Can you work these out from the drawing? Everything is in mm from the part's minimum corner. A direction names the side the tool comes from. Coordinates: 2 decimals unless noted, no trailing zeros. Loops run counter-clockwise (first coordinate to the right, second up) from the corner with the lowest first, then second, coordinate; pieces in that order, holes last.
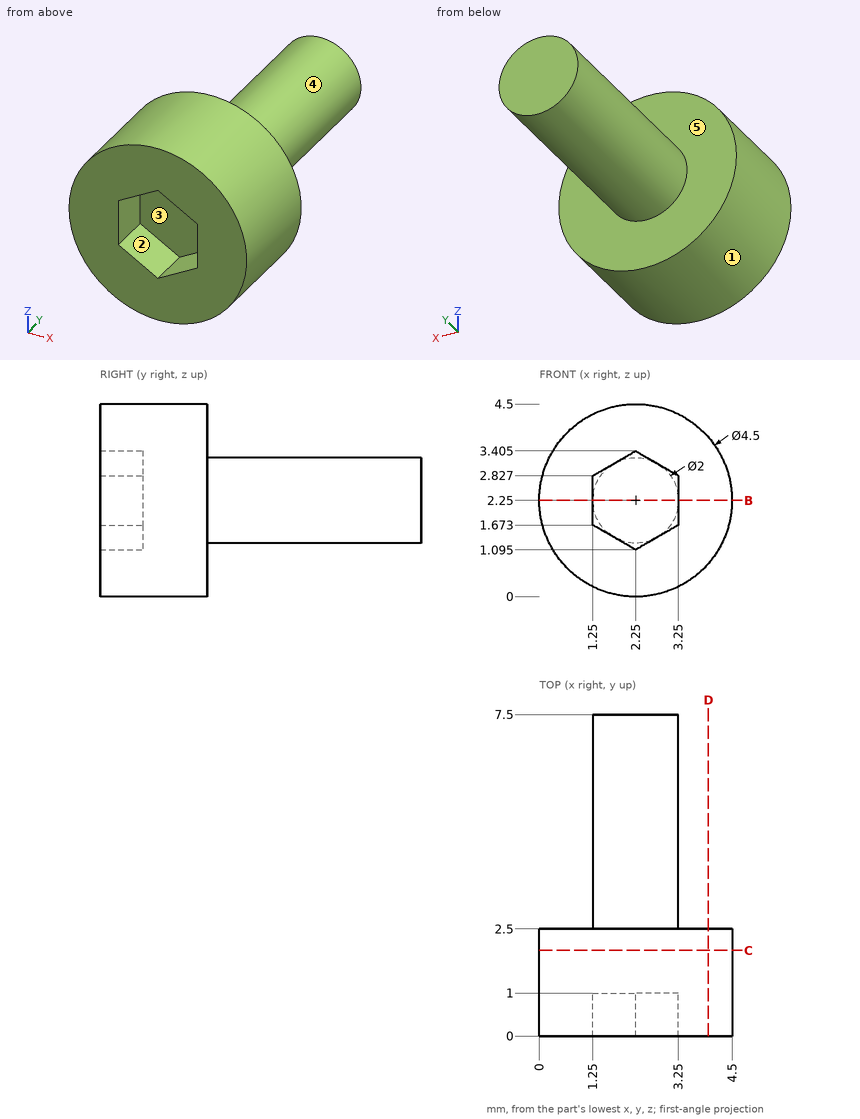
1. I want a section at D-D (x = 3.95). Please give me the cut outline in (y, z).
2. On a 3-axis mill with a long thin cutter (end or side, diameter ignored), from which of +Z, -Z, +X, -X, +Y, -Y can I reach the whole of each face in a straight line? I mean the marked faces 1 and 2. Say none if no direction works.
3. I want a section at B-B (z = 2.25). Please give me the cut outline in (x, y).
4. I want a section at C-C (y = 2). Please give me the cut outline in (x, z).
5. We'd pull the mould along Z, two halves only. Please class the marked faces 3, 4 and 5: +Z half, -Z half, draft (parallel to the pull), parting line (faces both ways), or undercut.
6. I need wall thicknesses on line 1 along Y through (x, z) = (3.35, 0.85); line 2 along Y through (x, z) = (3.05, 2.6); line 3 along Z through (x, y) = (3, 0.5). Which ranges of each line are inside material? Lowest first, please.
7. For pin 1 (0.6 mm diameter, centred on x = 2, z = 2.5, fed in from -Y), with a flat end and sliding along its axis, tell me the tip position at first contact or that it passes through.
Response values:
1. outline: (0, 0.78) - (2.5, 0.78) - (2.5, 3.72) - (0, 3.72) - close
2. face 1: +Y, -Y
2. face 2: -Y
3. outline: (0, 0) - (1.25, 0) - (1.25, 1) - (3.25, 1) - (3.25, 0) - (4.5, 0) - (4.5, 2.5) - (3.25, 2.5) - (3.25, 7.5) - (1.25, 7.5) - (1.25, 2.5) - (0, 2.5) - close
4. outline: circle Ø4.5 at (2.25, 2.25)
5. face 3: undercut
5. face 4: parting line
5. face 5: draft
6. line 1: y = 0 to 2.5
6. line 2: y = 1 to 7.5
6. line 3: z = 0.13 to 1.53, 2.97 to 4.37
7. pin 1: stops at y = 1
